For this review, use the dimensioned drawing (mm, ordinates from the lowest corner) and the shaded views. A direction names the side the tool comes from. Round coordinates to 2 decimals unless told otherwise and drop trailing zeros. Write each loop counter-clockwise with the first axis right and the second up, starting at its lowest first coordinate (ties: lowest second). Pieces come first, ordered by that corner, then holes. Notation, with made-up numbers: M 16,-20.75 L 52,-20.75 A20 cw 52,3.25 Z; hole C -1,24.5 d7. An arc over 180 degrees is marked long. Use CSV: the item, a comma, the result in double quotes.
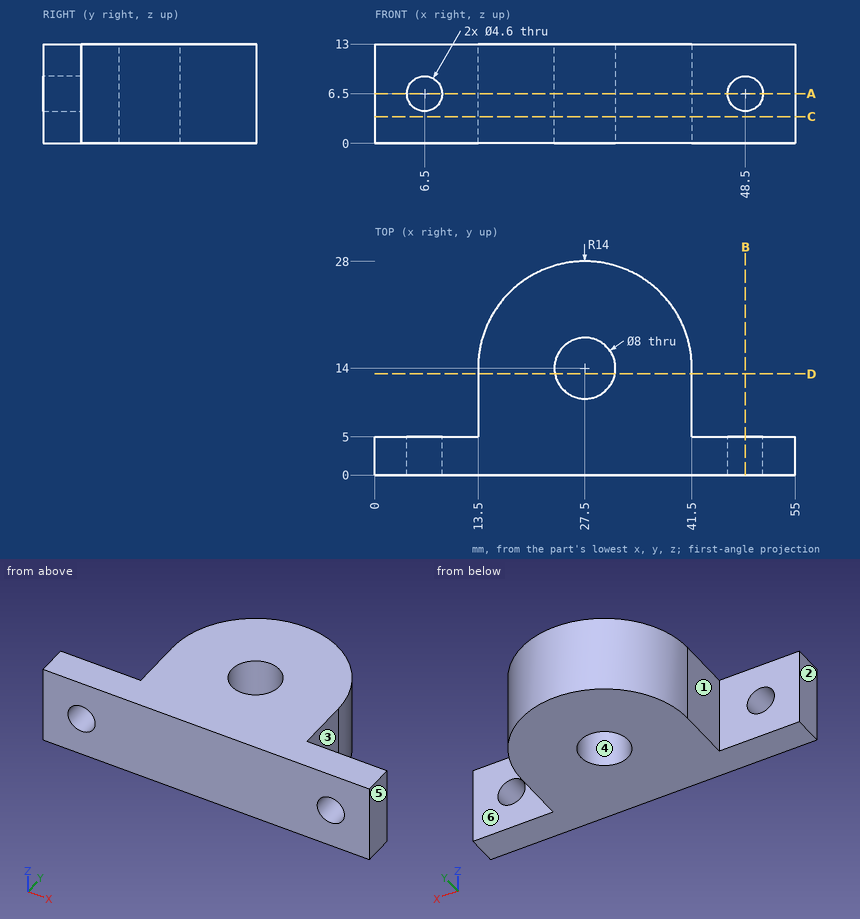
1) Add section A-A on z = 6.5. Write out the cut boundary in (x, y), then the cut area to 3 significant figures.
Answers:
outline,"M 0,0 L 4.2,0 L 4.2,5 L 0,5 Z; M 8.8,0 L 46.2,0 L 46.2,5 L 41.5,5 L 41.5,14 A14 ccw 13.5,14 L 13.5,5 L 8.8,5 Z; M 50.8,0 L 55,0 L 55,5 L 50.8,5 Z; hole C 27.5,14 d8"
area,"739 mm²"
2) For pin 1 Ø2 at (x, z) = (36.5, 2.5) entering from +Y; pin 2 Ø1.5 at (x, z) = (28.5, 11.5) entering from +Y; pin 3 Ø6 at (x, z) = (48.5, 6.5) entering from +Y, all flat-tipped, find the tip position at first contact; note any pin that passes through.
Answers:
pin 1,"y = 25.49"
pin 2,"y = 28"
pin 3,"y = 5"
3) Add section D-D on y = 13.25. Write out the cut boundary in (x, z).
Answers:
outline,"M 13.5,0 L 23.57,0 L 23.57,13 L 13.5,13 Z; M 31.43,0 L 41.5,0 L 41.5,13 L 31.43,13 Z"
4) Machinability: for the marked faces 1, 2 and 3, which of the approach directions +Z, -Z, +X, -X, +Y, -Y give a long, thin tool a straight path to every point of the face, cutting with its end or side? Answer none if there is none.
Answers:
face 1,"+Z, -Z, -X, +Y"
face 2,"+Z, -Z, -X, +Y, -Y"
face 3,"+Z, -Z, +X, +Y"
5) Add section C-C on z = 3.5. Write out the cut boundary in (x, y).
Answers:
outline,"M 0,0 L 55,0 L 55,5 L 41.5,5 L 41.5,14 A14 ccw 13.5,14 L 13.5,5 L 0,5 Z; hole C 27.5,14 d8"
6) Add section B-B on x = 48.5. Write out the cut boundary in (y, z), then the cut area to 3 significant figures.
Answers:
outline,"M 0,0 L 5,0 L 5,4.2 L 0,4.2 Z; M 0,8.8 L 5,8.8 L 5,13 L 0,13 Z"
area,"42.0 mm²"
7) Wall thickness on line 1 along X through (y, z) = (2.45, 6.5); line 2 along Y through (x, z) = (27.5, 9); line 3 along X through (y, z) = (4.75, 5.5): over which ranges is each line inside the solid? List them lowest first. Write a range as [from, to].
Answers:
line 1,"[0, 4.2], [8.8, 46.2], [50.8, 55]"
line 2,"[0, 10], [18, 28]"
line 3,"[0, 4.43], [8.57, 46.43], [50.57, 55]"
8) The part is to be moulded in two halves that separate along Y. For the marked faces 4, 5 and 6, say which applies: released by +Y, released by -Y, zero draft, split by the parting line, or undercut.
Answers:
face 4,"undercut"
face 5,"zero draft"
face 6,"released by +Y"
